```python
from build123d import *

# Parameters (mm, degrees)
F1_DEPTH      = 3
F3_DEPTH      = 50
F4_DEPTH      = 2
F5_R          = 65
F6_DEPTH      = 120.0131182079
F6_DEPTH_BACK = 70


with BuildPart() as f1:
    # F0 (on Top) → F1 (new body)
    with BuildSketch(Plane.XY):
        with BuildLine():
            ThreePointArc((-67.0229373247, 119.8506346331), (-67.6147835705, 104.9467461722), (-56.5, 95))
            ThreePointArc((-56.5, 95), (-51.5, 94.2705098312), (-46.5, 95))
            ThreePointArc((-46.5, 95), (-35.3852164295, 104.9467461722), (-35.9770626753, 119.8506346331))
            ThreePointArc((-35.9770626753, 119.8506346331), (-36.1592170528, 120.0001318772), (-36.3931701723, 119.971925829))
            Line((-36.3931701723, 119.971925829), (-38.0403835084, 119.020906766))
            ThreePointArc((-38.0403835084, 119.020906766), (-38.178168335, 118.8458333976), (-38.1572387337, 118.6240287662))
            ThreePointArc((-38.1572387337, 118.6240287662), (-51.5, 96.7705098312), (-64.8427612663, 118.6240287662))
            ThreePointArc((-64.8427612663, 118.6240287662), (-64.821831665, 118.8458333976), (-64.9596164916, 119.020906766))
            Line((-64.9596164916, 119.020906766), (-66.6068298277, 119.971925829))
            ThreePointArc((-66.6068298277, 119.971925829), (-66.8407829472, 120.0001318772), (-67.0229373247, 119.8506346331))
        make_face()
        with BuildLine():
            Line((-56.5, 95), (-56.5, 55))
            Line((-56.5, 55), (-46.5, 55))
            Line((-46.5, 55), (-46.5, 95))
            ThreePointArc((-46.5, 95), (-51.5, 94.2705098312), (-56.5, 95))
        make_face()
        with BuildLine():
            Line((46.5, 55), (56.5, 55))
            Line((56.5, 55), (56.5, 95))
            ThreePointArc((56.5, 95), (51.5, 94.2705098312), (46.5, 95))
            Line((46.5, 95), (46.5, 55))
        make_face()
        with BuildLine():
            Line((-88, -55), (88, -55))
            ThreePointArc((88, -55), (89.4142135624, -54.4142135624), (90, -53))
            Line((90, -53), (90, 53))
            ThreePointArc((90, 53), (89.4142135624, 54.4142135624), (88, 55))
            Line((88, 55), (56.5, 55))
            Line((56.5, 55), (46.5, 55))
            Line((46.5, 55), (-46.5, 55))
            Line((-46.5, 55), (-56.5, 55))
            Line((-56.5, 55), (-88, 55))
            ThreePointArc((-88, 55), (-89.4142135624, 54.4142135624), (-90, 53))
            Line((-90, 53), (-90, -53))
            ThreePointArc((-90, -53), (-89.4142135624, -54.4142135624), (-88, -55))
        make_face()
        with BuildLine():
            ThreePointArc((46.5, 95), (51.5, 94.2705098312), (56.5, 95))
            ThreePointArc((56.5, 95), (67.6147835705, 104.9467461722), (67.0229373247, 119.8506346331))
            ThreePointArc((67.0229373247, 119.8506346331), (66.8416372621, 119.999881477), (66.6083744282, 119.9728115034))
            Line((66.6083744282, 119.9728115034), (64.9559948815, 119.031841137))
            ThreePointArc((64.9559948815, 119.031841137), (64.8168865883, 118.8566295505), (64.837696354, 118.6338804295))
            ThreePointArc((64.837696354, 118.6338804295), (51.494682782, 96.7705107737), (38.1671728693, 118.6433346293))
            ThreePointArc((38.1671728693, 118.6433346293), (38.1878631933, 118.8669988874), (38.0474675348, 119.0423352753))
            Line((38.0474675348, 119.0423352753), (36.3900688241, 119.9735613901))
            ThreePointArc((36.3900688241, 119.9735613901), (36.157480746, 119.9995347637), (35.9770092024, 119.8505319041))
            ThreePointArc((35.9770092024, 119.8505319041), (35.385239009, 104.9466928494), (46.5, 95))
        make_face()
    extrude(amount=F1_DEPTH)

    # F2 (on face) → F3 (join)
    with BuildSketch(Plane.XY.offset(3)):
        with BuildLine():
            Line((-46.5, 55), (-56.5, 55))
            Line((-56.5, 55), (-88, 55))
            ThreePointArc((-88, 55), (-89.4142135624, 54.4142135624), (-90, 53))
            Line((-90, 53), (-90, -53))
            ThreePointArc((-90, -53), (-89.4142135624, -54.4142135624), (-88, -55))
            Line((-88, -55), (88, -55))
            ThreePointArc((88, -55), (89.4142135624, -54.4142135624), (90, -53))
            Line((90, -53), (90, 53))
            ThreePointArc((90, 53), (89.4142135624, 54.4142135624), (88, 55))
            Line((88, 55), (56.5, 55))
            Line((56.5, 55), (46.5, 55))
            Line((46.5, 55), (-46.5, 55))
        make_face()
        Polygon((-88, 53), (-56.5, 53), (-46.5, 53), (46.5, 53), (56.5, 53), (88, 53), (88, -53), (-88, -53), align=None, mode=Mode.SUBTRACT)
    extrude(amount=F3_DEPTH)

    # F4 (add): faces of the model
    f4_faces = [f1.faces().sort_by_distance(p)[0] for p in [
        (51.4996732425, 83.726401448, 3),
        (-51.5, 83.7238009637, 3),
    ]]
    extrude(f4_faces, amount=F4_DEPTH)

    # F5 (on Front) → F6 (cut, two sides)
    with BuildSketch(Plane.XZ) as f6_sk:
        with Locations((0, 185)):
            Circle(F5_R)
    extrude(amount=-F6_DEPTH, mode=Mode.SUBTRACT)
    extrude(f6_sk.sketch, amount=F6_DEPTH_BACK, mode=Mode.SUBTRACT)


solid = f1.part
```
Can you work these out from the model? Positions are in its coordinate system, mm. A direction names the side the tool comes from. Coordinates: 2 decimals unless noted, no trailing zeros. Write each loop counter-clockwise with the first axis right and the second up, starting at its lowest first coordinate (ties: lowest second). Pieces come first, ordered by that corner, then holes. Notation, with made-up numbers: M 73,68 L 110,68 A25 cw 110,106 Z; hole C 60.25,18.5 d9. An arc over 180 degrees is marked long. Answer as CSV lines item,"result".
Item 1: Imagine slicing it at C-C on x = -51.5. List the corners of the cut face in (y, z) for me.
Geometry results:
outline,"M -55,0 L 96.77,0 L 96.77,5 L 55,5 L 55,53 L 53,53 L 53,3 L -53,3 L -53,53 L -55,53 Z"
Item 2: We'd pull the mould along Y, two halves only. Please class faces 5 (the flat face through (-1, -55, 26)), 6 (the flat face through (-1, 53, 28)), 7 (the flat face through (-1, 14, 0)): +Y half, -Y half, draft (parallel to the pull), parting line (faces both ways), or undercut.
Geometry results:
face 5,"-Y half"
face 6,"undercut"
face 7,"draft"
Item 3: Imagine slicing it at D-D on y = 39. List the corners of the cut face in (x, z) for me.
Geometry results:
outline,"M -90,0 L 90,0 L 90,53 L 88,53 L 88,3 L -88,3 L -88,53 L -90,53 Z"
Item 4: Please list where these lines run through material, in increasing order: line 1 along X through (y, z) = (51.5, 44); line 2 along Y through (x, z) = (-51.5, 3.35); line 3 along Y through (x, z) = (-65.5, 48).
Geometry results:
line 1,"x = -90 to -88, 88 to 90"
line 2,"y = -55 to -53, 53 to 96.77"
line 3,"y = -55 to -53, 53 to 55"
Item 5: Imagine slicing it at B-B on z = 12.5. List the corners of the cut face in (x, y) for me, plus the area to 3 significant figures.
Geometry results:
outline,"M -90,-53 A2 ccw -88,-55 L 88,-55 A2 ccw 90,-53 L 90,53 A2 ccw 88,55 L -88,55 A2 ccw -90,53 Z; hole M -88,-53 L 88,-53 L 88,53 L -88,53 Z"
area,"1,140 mm2"
Item 6: On a 3-axis mill with a long thin cutter (end or side, diameter ignored), from which of +Z, -Z, +X, -X, +Y, -Y can I reach the whole of each face in a straight line? I mean faces 1 (the flat face through (-52, 85, 5)), 2 (the flat face through (-56.5, 75, 2)), 3 (the cylindrical face through (35.3, 105.15, 2.46)), 4 (the flat face through (1, -53, 28)). Say none if no direction works.
Geometry results:
face 1,"+Z, +X, -X, +Y"
face 2,"+Z, -Z, -X"
face 3,"+Z, -Z"
face 4,"+Z"
Item 7: Imagine slicing it at A-A on y = 70. List the corners of the cut face in (x, z) for me.
Geometry results:
outline,"M -56.5,0 L -46.5,0 L -46.5,5 L -56.5,5 Z; M 46.5,0 L 56.5,0 L 56.5,5 L 46.5,5 Z"
Item 8: I'm going to push flat-ended pins straight in: P1, Ø17.5, axis at x = 60, y = 80.5, coming from the +Z side; P2, Ø4, axis at y = 75.5, z = 3.5, coming from the +X side; P3, Ø1.5, axis at x = 4.5, y = 13, coming from the -Z side; P4, Ø3, axis at x = -46.5, z = 46.5, coming from the +Y side. Where does each tip first touch, or does it pass through?
Geometry results:
P1,"stops at z = 5"
P2,"stops at x = 56.5"
P3,"stops at z = 0"
P4,"stops at y = 55"
